Model file for the job. Use its own axes, mm. Give positions to 0.01 mm unless a question says otherwise; leave off trailing zeros. Order: outer loops, then holes, each group sorted by start corner. A loop starts at its lowest first (then second) coordinate and runs counter-clockwise, first axis right, second up. Notation, with made-up numbers: (82.25, 62.5) - (110.25, 62.5) arc R32 cw to (110.25, 99.5) - close; hole circle Ø11 at (23.25, -22.75). An arc over 180 degrees is marked (long way). Use CSV: the item, a comma, the result in double quotes. Start each with the question number.
(1) Pull direction Z, two halves, no side cores. Call faces 1 (the cylindrical face through (-11.19, -3.45, 0.49)), 2 (the flat face through (0, 0, -12)), 3 (the cylindrical face through (-12.85, -6.43, -23.83)): +Z half, -Z half, draft (parallel to the pull), parting line (faces both ways), or undercut.
(2) Band-saw the part on A-A, the plane y = -3.25. Give the cut face in (x, z).
(3) Drop flat-ended pins along their axis: pin 1 Ø2 at (x, y) = (-15.5, -1.5) entering from -Z; pin 2 Ø2 at (y, z) = (-1.5, 10) entering from +X; pin 3 Ø2 at (y, z) = (-5.5, 14) entering from +X. Give the stop position or say it passes through.
(4) Probe L1, parallel to Z at x = -7, y = -6.5; L2, parallel to Z at x = 0, y = -5; L3, parallel to X at y = -0.75, z = 14.5. List the from-to ranges inside material, lowest first.
from build123d import *

# Parameters (mm, degrees)
F0_R     = 13.2
F0_R_2   = 11.2
F1_DEPTH = 7
F2_R     = 2
F3_R     = 2


with BuildPart() as f1:
    # F0 (on Front) → F1 (new body)
    with BuildSketch(Plane.XZ):
        Polygon((18.775388, -23.340316), (29.7803, -3.227892), (23.340316, 18.775388), (3.227892, 29.7803), (-18.775388, 23.340316), (-29.7803, 3.227892), (-23.340316, -18.775388), (-3.227892, -29.7803), align=None)
        Circle(F0_R, mode=Mode.SUBTRACT)
        Circle(F0_R)
        Circle(F0_R_2, mode=Mode.SUBTRACT)
    extrude(amount=F1_DEPTH)

    # F2
    f2_edges = [f1.edges().sort_by_distance(p)[0] for p in [
        (13.284104, 0, 24.277844),
        (26.560308, 0, 7.773748),
        (24.277844, 0, -13.284104),
        (7.773748, 0, -26.560308),
        (-13.284104, 0, -24.277844),
        (-26.560308, 0, -7.773748),
        (-24.277844, 0, 13.284104),
        (-7.773748, 0, 26.560308),
    ]]
    fillet(f2_edges, radius=F2_R)

    # F3
    f3_edges = [f1.edges().sort_by_distance(p)[0] for p in [
        (-7.773748, -7, 26.560308),
        (-24.277844, -7, 13.284104),
        (-26.560308, -7, -7.773748),
        (-13.284104, -7, -24.277844),
        (7.773748, -7, -26.560308),
        (24.277844, -7, -13.284104),
        (26.560308, -7, 7.773748),
        (13.284104, -7, 24.277844),
    ]]
    fillet(f3_edges, radius=F3_R)


solid = f1.part
Answer block:
1,face 1,"undercut"
1,face 2,"draft"
1,face 3,"-Z half"
2,outline,"(-29.78, 3.23) - (-23.34, -18.78) - (-3.23, -29.78) - (18.78, -23.34) - (29.78, -3.23) - (23.34, 18.78) - (3.23, 29.78) - (-18.78, 23.34) - close; hole circle Ø22.4 at (0, 0)"
3,pin 1,"stops at z = -23.58"
3,pin 2,"stops at x = 26.18"
3,pin 3,"stops at x = 25.01"
4,L1,"z = -26.94 to -8.74, 8.74 to 26.08"
4,L2,"z = -28.84 to -11.2, 11.2 to 28.84"
4,L3,"x = -23.11 to 24.13"
